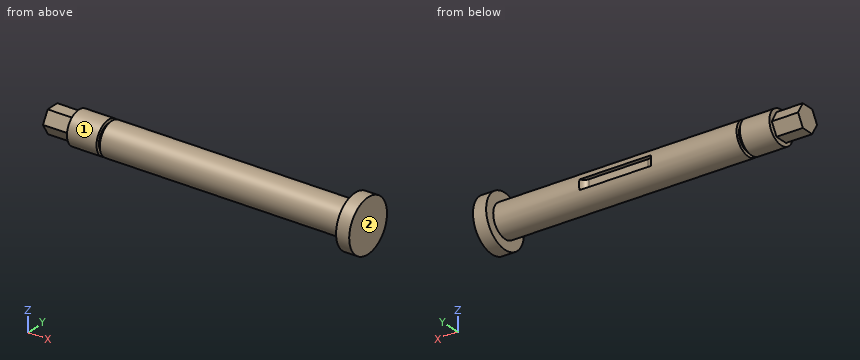
```python
from build123d import *

# Parameters (mm, degrees)
CUT_EXTRUDE1_DEPTH = 2.38125
SKETCH6_OUTSIDE_W  = 58.716
SKETCH6_OUTSIDE_H  = 58.716
CUT_EXTRUDE2_DEPTH = 12.7


with BuildPart() as part:
    # Sketch2 → Revolve1 (revolve)
    with BuildSketch(Plane.XY, mode=Mode.PRIVATE) as revolve1_sk:
        Polygon((0, 0), (0, 6.35), (12.7, 6.35), (12.7, 7.9375), (26.9748, 7.9375), (26.9748, 6.3373), (28.575, 6.3373), (28.575, 7.9375), (146.05, 7.9375), (146.05, 12.7), (152.4, 12.7), (152.4, 0), align=None)
    revolve(revolve1_sk.sketch.rotate(Axis((-160.725070543, 0, 0), (1, 0, 0)), 90), axis=Axis((-160.725070543, 0, 0), (1, 0, 0)))

    # Sketch3 → Cut-Extrude1 (cut, symmetric)
    with BuildSketch(Plane.XY):
        with BuildLine():
            Line((69.85, 14.2875), (104.775, 14.2875))
            Line((104.775, 14.2875), (104.775, 8.7249))
            ThreePointArc((104.775, 8.7249), (103.84506403, 6.47983597), (101.6, 5.5499))
            Line((101.6, 5.5499), (73.025, 5.5499))
            ThreePointArc((73.025, 5.5499), (70.77993597, 6.47983597), (69.85, 8.7249))
            Line((69.85, 8.7249), (69.85, 14.2875))
        make_face()
    extrude(amount=CUT_EXTRUDE1_DEPTH, both=True, mode=Mode.SUBTRACT)

    # Sketch6 outside → Cut-Extrude2 (cut)
    with BuildSketch(Plane.ZY):
        Rectangle(SKETCH6_OUTSIDE_W, SKETCH6_OUTSIDE_H)
        Polygon((0, 6.35), (-5.499261314, 3.175), (-5.499261314, -3.175), (0, -6.35), (5.499261314, -3.175), (5.499261314, 3.175), align=None, mode=Mode.SUBTRACT)
    extrude(amount=-CUT_EXTRUDE2_DEPTH, mode=Mode.SUBTRACT)


solid = part.part
```
CAD build for the part. Positions are in the model's coordinates, mm. Face numbers are marked on the shaded views. Give positions to 0.01 mm unless a question says otherwise; leave off trailing zeros. Write each loop counter-clockwise with the first axis right and the second up, starting at its lowest first coordinate (ties: lowest second). Pieces come first, ordered by that corner, then holes. Notation, with made-up numbers: M 17,87.25 L 65,87.25 A20 ccw 65,101.25 Z; hole C -7.75,34 d1. An arc over 180 degrees is marked long. Return JSON: item names as keys, results as strings. Group by question number.
(1) Band-saw the part on D-D (z = 9.5). Give the cut face in (x, y).
(2) Band-saw the part on C-C (x = 90). Give the cut face in (y, z) (1 decimal).
(3) Flat gauge pins, fed straight in: pin 1 Ø1 at (x, z) = (39.5, -2) entering from -Y; pin 2 Ø2 at (x, y) = (87.5, 6.5) entering from +Z; pin 3 Ø2 at (x, y) = (79, 7) entering from -Z. Where does each tip first touch, or does it go through?
(4) Mould opens along Y. For the marked faces 1 and 2 say: pulls with the +Y half, pulls with the -Y half, needs draft (parallel to the pull), parting line crosses it, or undercut.
(5) Drill centre lines: L1, parallel to X at y = 2.75, z = 9.25; L2, parallel to Z at x = 46, y = -5.75; L3, parallel to Z at x = 124, y = 2.25. Where is each one in solid material? Low to high. Write a range as [from, to].
(6) Band-saw the part on B-B (x = 11). Give the cut face in (y, z) (3 decimals), and give its area (3 significant figures).
Entries:
{
 "1": {"outline": "M 146.05,-8.43 L 152.4,-8.43 L 152.4,8.43 L 146.05,8.43 Z"},
 "2": {"outline": "M 5.5,-2.4 L 5.5,2.4 L 7.6,2.4 A7.9 ccw long 7.6,-2.4 Z"},
 "3": {"pin 1": "stops at y = -7.79", "pin 2": "stops at z = 5.72", "pin 3": "stops at z = -5.2"},
 "4": {"face 1": "parting line crosses it", "face 2": "needs draft"},
 "5": {"L1": "x = [146.05, 152.4]", "L2": "z = [-5.47, 5.47]", "L3": "z = [-7.61, 7.61]"},
 "6": {"outline": "M -6.35,0 L -3.175,-5.499 L 3.175,-5.499 L 6.35,0 L 3.175,5.499 L -3.175,5.499 Z", "area": "105 mm^2"}
}
